For this review, take the finished solid that the model builds, in its own axes (mm). A direction names the side the tool comes from. Round coordinates to 2 decimals unless told otherwise and drop trailing zeros. Write each loop counter-clockwise with the first axis right and the second up, starting at its lowest first coordinate (ties: lowest second). Pieces come first, ordered by that corner, then holes. Notation, with made-up numbers: M 61,26 L 74,26 A22 cw 74,54 Z; hole C 89,86.25 d5. An arc over 180 degrees is marked long. Use one line per item in the form item = value. Start each with the question number.
Item 1: Add section D-D (x = 1.5). State the section outline as (y, z) points, and give its area (4 significant figures).
Item 2: Add section B-B (x = -33.5). State the section outline as (y, z) points, and give its area (3 significant figures).
Item 3: Draft analysis for pull direction Z (two halves, no side actions). For faces 1 (the cylindrical face through (-33.979, 0.507, -18.595)), 2 (the flat face through (0, 2, -19.25)), 3 (the flat face through (0, 0, 0)), 4 (the cylindrical face through (-33.979, 0.507, 20.905)), state which applies: released by +Z, released by -Z, zero draft, split by the parting line, or undercut.
Item 4: Add section A-A (z = 19.75). State the section outline as (x, y) points, and give its area (3 significant figures).
Item 5: Add section C-C (z = -14). State the section outline as (x, y) points, and give its area (3 significant figures).
Item 6: For line 1 (X direction, y = 0.75, z = 19.75); line 2 (X direction, y = 2.05, z = -18); line 3 (Z direction, x = 8.5, y = 2.3), list the stretches that pass through material, from the lowest coordinate up. Write a range as [from, to].
Item 7: For P1, Ø5, axis at x = -26, z = 14.5, coming from the -Y side; P2, Ø3, axis at x = 33.5, z = -19.75, coming from the +Y side; P3, Ø0.9, axis at y = 2, z = -8.5, coming from the -X side; P4, Ø0.9, axis at x = -2.5, y = 2, coming from the -Z side, all flat-tipped, find the tip position at first contact; note any pin that passes through.
Item 8: For faces 5 (the flat face through (31.5, 2, 2)), 6 (the flat face through (0, 2, 21.75)), 7 (the flat face through (-31.5, 2, 2)), list the 3-axis set-ups (+Z, -Z, +X, -X, +Y, -Y) from which the entire face can be reached by the end or side of a thin tool; tool diameter is ignored.
from build123d import *

# Parameters (mm, degrees)
SKETCH_1_W          = 71
SKETCH_1_H          = 43.5
EXTRUDE_1_DEPTH     = 1
CUT_EXTRUDE_1_REACH = 43.645
SKETCH_6_R          = 1.25
SKETCH_4_W          = 63
SKETCH_4_H          = 41
EXTRUDE_2_DEPTH     = 3


with BuildPart() as part:
    # 草图1 → 凸台-拉伸1 (new body)
    with BuildSketch(Plane(origin=(0, 0, 0), x_dir=(1, 0, 0), z_dir=(0, 1, 0))):
        Rectangle(SKETCH_1_W, SKETCH_1_H)
    extrude(amount=EXTRUDE_1_DEPTH)

    # 草图6 → 切除-拉伸1 (cut, up to next)
    with BuildSketch(Plane(origin=(0, 1, 0), x_dir=(1, 0, 0), z_dir=(0, 1, 0)), mode=Mode.PRIVATE) as cut_extrude_1_sk1:
        with Locations(Location((-33.5, 19.75, 0), (0, 0, 270))):
            Circle(SKETCH_6_R)
    cut_extrude_1_tool1 = extrude(cut_extrude_1_sk1.sketch, amount=-CUT_EXTRUDE_1_REACH, mode=Mode.PRIVATE) & part.part
    # 草图6 → 切除-拉伸1 (cut, up to next)
    with BuildSketch(Plane(origin=(0, 1, 0), x_dir=(1, 0, 0), z_dir=(0, 1, 0)), mode=Mode.PRIVATE) as cut_extrude_1_sk2:
        with Locations(Location((33.5, 19.75, 0), (0, 0, 270))):
            Circle(SKETCH_6_R)
    cut_extrude_1_tool2 = extrude(cut_extrude_1_sk2.sketch, amount=-CUT_EXTRUDE_1_REACH, mode=Mode.PRIVATE) & part.part
    # 草图6 → 切除-拉伸1 (cut, up to next)
    with BuildSketch(Plane(origin=(0, 1, 0), x_dir=(1, 0, 0), z_dir=(0, 1, 0)), mode=Mode.PRIVATE) as cut_extrude_1_sk3:
        with Locations(Location((33.5, -19.75, 0), (0, 0, 270))):
            Circle(SKETCH_6_R)
    cut_extrude_1_tool3 = extrude(cut_extrude_1_sk3.sketch, amount=-CUT_EXTRUDE_1_REACH, mode=Mode.PRIVATE) & part.part
    # 草图6 → 切除-拉伸1 (cut, up to next)
    with BuildSketch(Plane(origin=(0, 1, 0), x_dir=(1, 0, 0), z_dir=(0, 1, 0)), mode=Mode.PRIVATE) as cut_extrude_1_sk4:
        with Locations(Location((-33.5, -19.75, 0), (0, 0, 270))):
            Circle(SKETCH_6_R)
    cut_extrude_1_tool4 = extrude(cut_extrude_1_sk4.sketch, amount=-CUT_EXTRUDE_1_REACH, mode=Mode.PRIVATE) & part.part
    add(cut_extrude_1_tool1.solids().sort_by_distance((-33.5, 1, -19.75))[0], mode=Mode.SUBTRACT)
    add(cut_extrude_1_tool2.solids().sort_by_distance((33.5, 1, -19.75))[0], mode=Mode.SUBTRACT)
    add(cut_extrude_1_tool3.solids().sort_by_distance((33.5, 1, 19.75))[0], mode=Mode.SUBTRACT)
    add(cut_extrude_1_tool4.solids().sort_by_distance((-33.5, 1, 19.75))[0], mode=Mode.SUBTRACT)

    # 草图4 → 凸台-拉伸2 (add)
    with BuildSketch(Plane(origin=(0, 1, 0), x_dir=(1, 0, 0), z_dir=(0, 1, 0))):
        with Locations((0, -1.25)):
            Rectangle(SKETCH_4_W, SKETCH_4_H)
    extrude(amount=EXTRUDE_2_DEPTH)


solid = part.part
Calculated:
q1.outline = M 0,-21.75 L 1,-21.75 L 1,-19.25 L 4,-19.25 L 4,21.75 L 0,21.75 Z
q1.area = 166.5 mm^2
q2.outline = M 0,-21.75 L 1,-21.75 L 1,-21 L 0,-21 Z; M 0,-18.5 L 1,-18.5 L 1,18.5 L 0,18.5 Z; M 0,21 L 1,21 L 1,21.75 L 0,21.75 Z
q2.area = 38.5 mm^2
q3.face_1 = undercut
q3.face_2 = released by -Z
q3.face_3 = zero draft
q3.face_4 = undercut
q4.outline = M -35.5,0 L -34.75,0 L -34.75,1 L -35.5,1 Z; M -32.25,0 L 32.25,0 L 32.25,1 L 31.5,1 L 31.5,4 L -31.5,4 L -31.5,1 L -32.25,1 Z; M 34.75,0 L 35.5,0 L 35.5,1 L 34.75,1 Z
q4.area = 255 mm^2
q5.outline = M -35.5,0 L 35.5,0 L 35.5,1 L 31.5,1 L 31.5,4 L -31.5,4 L -31.5,1 L -35.5,1 Z
q5.area = 260 mm^2
q6.line_1 = [-35.5, -34.75], [-32.25, 32.25], [34.75, 35.5]
q6.line_2 = [-31.5, 31.5]
q6.line_3 = [-19.25, 21.75]
q7.P1 = 0
q7.P2 = 1
q7.P3 = -31.5
q7.P4 = -19.25
q8.face_5 = +Z, -Z, +X, +Y
q8.face_6 = +Z, +X, -X, +Y, -Y
q8.face_7 = +Z, -Z, -X, +Y
